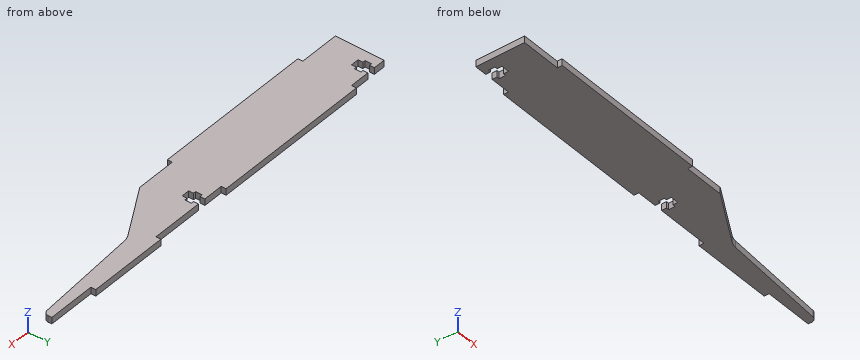
```python
from build123d import *

# Parameters (mm, degrees)
SKETCH1_W           = 150
SKETCH1_H           = 30
SKETCH1_W_2         = 100
SKETCH1_H_2         = 6
BOSS_EXTRUDE1_DEPTH = 4
SKETCH2_W           = 5
SKETCH2_H           = 20
SKETCH2_W_2         = 8.2
SKETCH2_H_2         = 4
CUT_EXTRUDE1_DEPTH  = 10
SKETCH3_W           = 50
SKETCH3_H           = 3
BOSS_EXTRUDE2_DEPTH = 4


with BuildPart() as part:
    # Sketch1 → Boss-Extrude1 (new body)
    with BuildSketch(Plane.XY):
        Rectangle(SKETCH1_W, SKETCH1_H)
        with Locations((0, -15)):
            Rectangle(SKETCH1_W_2, SKETCH1_H_2)
        with Locations((0, 15)):
            Rectangle(SKETCH1_W_2, SKETCH1_H_2)
    extrude(amount=BOSS_EXTRUDE1_DEPTH)

    # Sketch2 → Cut-Extrude1 (cut)
    with BuildSketch(Plane.XY.offset(4)):
        with Locations((-65, 15)):
            Rectangle(SKETCH2_W, SKETCH2_H)
        with Locations((-65, 10)):
            Rectangle(SKETCH2_W_2, SKETCH2_H_2)
    cut_extrude1 = extrude(amount=-CUT_EXTRUDE1_DEPTH, mode=Mode.SUBTRACT)

    # Mirror1: Cut-Extrude1 across plane
    add(cut_extrude1.mirror(Plane(origin=(0, 0, 0), x_dir=(0, 0, 1), z_dir=(1, 0, 0))), mode=Mode.SUBTRACT)

    # Sketch3 → Boss-Extrude2 (add)
    with BuildSketch(Plane.XY.offset(4)):
        with BuildLine():
            ThreePointArc((180, 12.794373235), (179.195218474, 10.749619986), (177.212656099, 9.80191983))
            Line((177.212656099, 9.80191983), (111.937946201, 5.163229336))
            ThreePointArc((111.937946201, 5.163229336), (109.717672062, 4.749776304), (107.646799864, 3.84863869))
            Line((107.646799864, 3.84863869), (75, -15))
            Line((75, -15), (75, 15))
            Line((75, 15), (180, 15))
            Line((180, 15), (180, 12.794373235))
        make_face()
        with Locations((125, 16.5)):
            Rectangle(SKETCH3_W, SKETCH3_H)
    extrude(amount=-BOSS_EXTRUDE2_DEPTH)


solid = part.part
```
Geometry: final body of the model. Coordinates: model frame, mm. Round coordinates to 2 decimals unless told otherwise and drop trailing zeros. Order: outer loops, then holes, each group sorted by start corner. A loop starts at its lowest first (then second) coordinate and runs counter-clockwise, first axis right, second up. Notation, with made-up numbers: M 39.25,55 L 54.25,55 A30 cw 54.25,92 Z; hole C 79.5,37 d1. An arc over 180 degrees is marked long. Use one line per item in the form item = value. Start each with the question number.
Q1. Pin query (flat end, axial travel): pin 1 Ø1.5 at (y, z) = (-3, 2.5) entering from +X; pin 2 Ø2 at (x, z) = (-64, 3) entering from +Y; pin 3 Ø0.9 at (y, z) = (17, 3) entering from +X. Return the tip coordinate at first contact, or that it passes through.
Q2. Cut plane B-B (y = -4). Return loops of the section in (x, z), and give its area (3 significant figures).
Q3. Material intervals for line 1 (X direction, y = 13, z = 1.3); line 2 (X direction, y = 16, z = 3.1); line 3 (X direction, y = -16, z = 1.2), sorted ascending. Write a range as [from, to].
Q4. Cut plane A-A (x = 58). Return loops of the section in (y, z).
Geometry results:
q1.pin_1 = 97.08
q1.pin_2 = 5
q1.pin_3 = 150
q2.outline = M -75,0 L 94.05,0 L 94.05,4 L -75,4 Z
q2.area = 676 mm^2
q3.line_1 = [-75, -67.5], [-62.5, 62.5], [67.5, 180]
q3.line_2 = [-50, 50], [100, 150]
q3.line_3 = [-50, 50]
q4.outline = M -15,0 L 15,0 L 15,4 L -15,4 Z
